Geometry: final body of the model. Coordinates: model frame, mm. A direction names the side the tool comes from. Round coordinates to 2 decimals unless told otherwise and drop trailing zeros. Loops run counter-clockwise (first coordinate to the right, second up) from the corner with the lowest first, then second, coordinate; pieces in that order, holes last. Notation, with made-up numbers: M 21,17.5 L 31,17.5 A8 ccw 31,30.5 Z; hole C 30,-33 d1. An arc over 180 degrees is marked long. Return JSON: item names as keys, results as strings.
from build123d import *

# Parameters (mm, degrees)
SKETCH1_R             = 2.5
BOSS_EXTRUDE1_DEPTH   = 10
BOSS_EXTRUDE1_2_DEPTH = 10
BOSS_EXTRUDE2_DEPTH   = 3
SKETCH3_R             = 0.8125
CUT_EXTRUDE1_DEPTH    = 20
CHAMFER1_SIZE         = 0.8
SKETCH4_R             = 3
BOSS_EXTRUDE3_DEPTH   = 10
CHAMFER2_SIZE         = 0.8
SKETCH5_R             = 0.8125
CUT_EXTRUDE2_DEPTH    = 20


with BuildPart() as part:
    # Sketch1 → Boss-Extrude1 (new body)
    with BuildSketch(Plane(origin=(0, 0, 0), x_dir=(0, 1, 0), z_dir=(0, 0, 1))):
        with Locations((-35, 0)):
            Circle(SKETCH1_R)
    extrude(amount=BOSS_EXTRUDE1_DEPTH)



with BuildPart() as body_2:
    # Sketch1 → Boss-Extrude1 2 (new body)
    with BuildSketch(Plane(origin=(0, 0, 0), x_dir=(0, 1, 0), z_dir=(0, 0, 1))):
        with Locations((35, 0)):
            Circle(SKETCH1_R)
    extrude(amount=BOSS_EXTRUDE1_2_DEPTH)


with BuildPart() as part_1:
    add(part.part)

    add(body_2.part)  # Boss-Extrude2 merges body 2
    # Sketch2 → Boss-Extrude2 (add)
    with BuildSketch(Plane(origin=(0, 0, 0), x_dir=(1, 0, 0), z_dir=(0, 0, -1))):
        with BuildLine():
            Line((4.5, 35), (4.5, -35))
            ThreePointArc((4.5, -35), (0, -39.5), (-4.5, -35))
            Line((-4.5, -35), (-4.5, 35))
            ThreePointArc((-4.5, 35), (0, 39.5), (4.5, 35))
        make_face()
    extrude(amount=BOSS_EXTRUDE2_DEPTH)

    # Sketch3 → Cut-Extrude1 (cut)
    with BuildSketch(Plane.XY.offset(10)):
        with Locations((0, -35)):
            Circle(SKETCH3_R)
        with Locations((0, 35)):
            Circle(SKETCH3_R)
    extrude(amount=-CUT_EXTRUDE1_DEPTH, mode=Mode.SUBTRACT)

    # Chamfer1
    chamfer1_edges = [part_1.edges().sort_by_distance(p)[0] for p in [
        (0, 32.5, 0),
        (0, -37.5, 0),
    ]]
    chamfer(chamfer1_edges, length=CHAMFER1_SIZE)

    # Sketch4 → Boss-Extrude3 (add)
    with BuildSketch(Plane.XY):
        with Locations(Location((0, 0, 0), (0, 0, 180))):
            Circle(SKETCH4_R)
    extrude(amount=BOSS_EXTRUDE3_DEPTH)

    # Chamfer2
    chamfer2_edges = [part_1.edges().sort_by_distance(p)[0] for p in [
        (3, 0, 0),
    ]]
    chamfer(chamfer2_edges, length=CHAMFER2_SIZE)

    # Sketch5 → Cut-Extrude2 (cut)
    with BuildSketch(Plane.XY.offset(10)):
        Circle(SKETCH5_R)
    extrude(amount=-CUT_EXTRUDE2_DEPTH, mode=Mode.SUBTRACT)


solid = part_1.part
Q1. Section query C-C (x = 0). State how many separate pieces and enclosed holes the cut face has, plus the area to 3 significant figures.
Determined:
{"separate pieces": "4", "enclosed holes": "0", "area": "336 mm^2"}
Q2. Section query B-B (y = 0). Output: boundary loops of the cut face in (x, z).
Determined:
{"outline": "M -4.5,-3 L -0.81,-3 L -0.81,10 L -3,10 L -3,0.8 L -3.8,0 L -4.5,0 Z; M 0.81,-3 L 4.5,-3 L 4.5,0 L 3.8,0 L 3,0.8 L 3,10 L 0.81,10 Z"}
Q3. Pin query (flat end, axial travel): pin 1 (4 mm diameter, centred on x = 3, z = -1, fed in from +Y); pin 2 (5 mm diameter, centred on x = -3.5, z = 4, fed in from -Y); pin 3 (2 mm diameter, centred on x = 0, y = 35, fed in from +Z); pin 4 (3 mm diameter, centred on x = -2, z = 4.5, fed in from -Y). Return the tip coordinate at first contact, or that it passes through.
Determined:
{"pin 1": "stops at y = 39.39", "pin 2": "stops at y = -37.29", "pin 3": "stops at z = 10", "pin 4": "stops at y = -37.45"}
Q4. Section query D-D (y = -29). Output: boundary loops of the cut face in (x, z), plus the area to 3 significant figures.
Determined:
{"outline": "M -4.5,-3 L 4.5,-3 L 4.5,0 L -4.5,0 Z", "area": "27.0 mm^2"}
Q5. Section query A-A (z = 8). Output: boundary loops of the cut face in (x, y) (1 decimal), plus the area to 3 significant figures.
Determined:
{"outline": "C 0,0 d6; C 0,-35 d5; C 0,35 d5; hole C 0,-35 d1.6; hole C 0,0 d1.6; hole C 0,35 d1.6", "area": "61.3 mm^2"}
Q6. Pull-direction query (Y, two-part tool) for faces 1 (the cylindrical face through (0.1, 39.5, -1.5)), 2 (the flat face through (-1, -36, 10)), 3 (the cylindrical face through (-0.645, -0.494, 3.591)); classes: pulls with the +Y half, pulls with the -Y half, needs draft (parallel to the pull), parting line crosses it, or undercut.
Determined:
{"face 1": "pulls with the +Y half", "face 2": "needs draft", "face 3": "undercut"}
Q7. Reachability of faces 4 (the cylindrical face through (-2.86, -0.9, 5.34)), 5 (the cylindrical face through (0.375, 34.279, 3.591)) from +Z, -Z, +X, -X, +Y, -Y: full face, straight path, thin tool, end or side. Return the list, or none.
Determined:
{"face 4": "+Z", "face 5": "+Z, -Z"}
Q8. Material intervals for L1, parallel to Y at x = 0, z = -0.25; L2, parallel to Y at x = 0, z = 5.25; L3, parallel to Z at x = -3.5, y = -23, sorted ascending.
Determined:
{"L1": "y = -39.5 to -35.81, -34.19 to -0.81, 0.81 to 34.19, 35.81 to 39.5", "L2": "y = -37.5 to -35.81, -34.19 to -32.5, -3 to -0.81, 0.81 to 3, 32.5 to 34.19, 35.81 to 37.5", "L3": "z = -3 to 0"}
